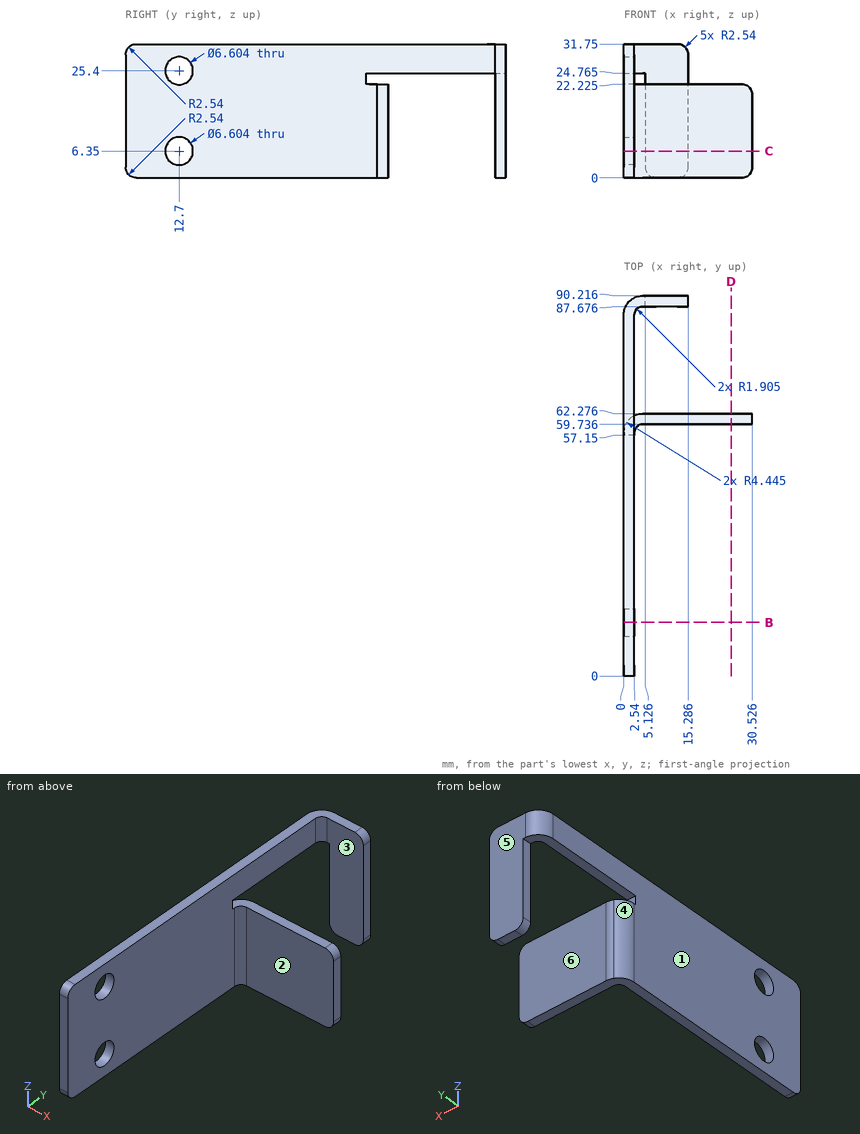
Design review of the part shown in the three views and the two pictorial views. Dimensions are in mm from the part's minimum x, y and z. A direction names the side the tool comes from. Give positions to 0.01 mm unless a question says otherwise; leave off trailing zeros. Write each loop counter-clockwise with the first axis right and the second up, starting at its lowest first coordinate (ties: lowest second). Pieces come first, ordered by that corner, then holes. Notation, with made-up numbers: M 14,12.25 L 35,12.25 A13 ccw 35,18.25 Z; hole C -32.5,-16.5 d9. An arc over 180 degrees is marked long. One line per item, written item: value.
1) The part is to be moulded in two halves that separate along Y. For the marked faces 1, 2 and 3, say which applies: +Y half, -Y half, draft (parallel to the pull), parting line (faces both ways), or undercut.
Results are:
face 1: draft
face 2: -Y half
face 3: undercut
2) For line 1 (Y direction, x = 14.5, z = 3); line 2 (X direction, y = 70, z = 26.5); line 3 (Y direction, x = 26.5, z = 14.5), list the stretches that pass through material, from the lowest coordinate up. Write a range as from..to.
Results are:
line 1: y = 59.74..62.28, 87.68..90.22
line 2: x = 0..2.54
line 3: y = 59.74..62.28
3) Take a section at D-D, the plane x = 25.5. Write out the cut boundary in (y, z) (1 decimal).
Results are:
outline: M 59.7,0 L 62.3,0 L 62.3,22.2 L 59.7,22.2 Z
4) For P1, Ø1.5, axis at x = 2.5, y = 71, coming from the -Z side (3 decimals); P2, Ø8, axis at y = 80, z = 11.5, coming from the -X side; P3, Ø12, axis at x = 11.5, z = 21.5, coming from the -Y side; P4, Ø2, axis at y = 89, z = 10.5, coming from the +X side, all flat-tipped, find the tip position at first contact; note any pin that passes through.
Results are:
P1: stops at z = 24.765
P2: passes through
P3: stops at y = 59.74
P4: stops at x = 15.29
5) For the marked faces 4, 5 and 6, list the 3-axis set-ups (+Z, -Z, +X, -X, +Y, -Y) from which the entire face can be reached by the end or side of a thin tool; tool diameter is ignored.
Results are:
face 4: -Z, -X, +Y
face 5: +Z, -Z, +X, -X, +Y
face 6: +Z, -Z, +X, -X
6) Take a section at C-C, the plane z = 6.35. Count the separate pieces of the cut face and the enclosed holes in it, then the cut area to 3 significant figures.
Results are:
separate pieces: 3
enclosed holes: 0
area: 235 mm²
7) Take a section at B-B, the plane y = 12.7. Write out the cut boundary in (x, z), then the cut area to 3 significant figures.
Results are:
outline: M 0,0 L 2.54,0 L 2.54,3.05 L 0,3.05 Z; M 0,9.65 L 2.54,9.65 L 2.54,22.1 L 0,22.1 Z; M 0,28.7 L 2.54,28.7 L 2.54,31.75 L 0,31.75 Z
area: 47.1 mm²
